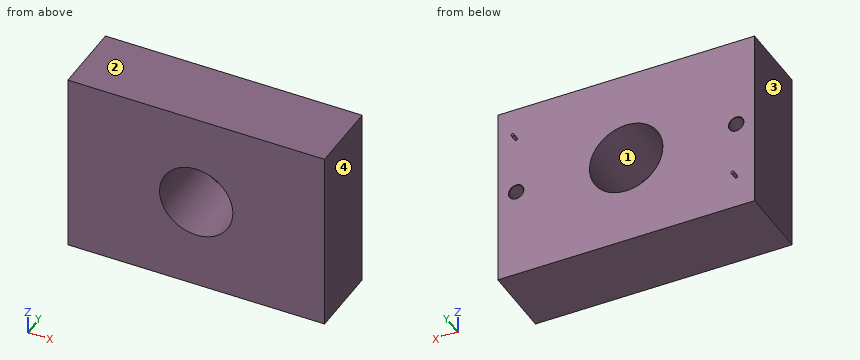
from build123d import *

# Parameters (mm, degrees)
SKETCH1_W                                      = 175
SKETCH1_H                                      = 125
SKETCH1_R                                      = 25
BOSS_EXTRUDE1_DEPTH                            = 50
SKETCH1_4_R                                    = 1
BOSS_EXTRUDE2_DEPTH                            = 5
CBORE_FOR_M12_HEX_HEAD_MACHINE_SCREW1_AT_COUNT = 2
CBORE_FOR_M12_HEX_HEAD_MACHINE_SCREW1_AT_PITCH = 150


with BuildPart() as part:
    # Sketch1 → Boss-Extrude1 (new body)
    with BuildSketch(Plane(origin=(0, 0, 0), x_dir=(1, 0, 0), z_dir=(0, 1, 0))):
        with Locations((87.5, 62.5)):
            Rectangle(SKETCH1_W, SKETCH1_H)
        with Locations(Location((87.5, 62.5, 0), (0, 0, 270))):
            Circle(SKETCH1_R, mode=Mode.SUBTRACT)
    extrude(amount=-BOSS_EXTRUDE1_DEPTH)

    # Sketch1_4 → Boss-Extrude2 (add)
    with BuildSketch(Plane(origin=(0, 0, 0), x_dir=(1, 0, 0), z_dir=(0, 1, 0))):
        with Locations(Location((12.5, 102.5, 0), (0, 0, 270))):
            Circle(SKETCH1_4_R)
        with Locations(Location((162.5, 22.5, 0), (0, 0, 270))):
            Circle(SKETCH1_4_R)
    extrude(amount=BOSS_EXTRUDE2_DEPTH)

    # Sketch5 → CBORE for M12 Hex Head Machine Screw1 (revolve, cut)
    with BuildSketch(Plane(origin=(12.5, 0, -62.5), x_dir=(0, 0, 1), z_dir=(1, 0, 0))):
        Polygon((0, 0), (0, 28), (4.25, 25.446342369), (4.25, 20), (5, 20), (5, 0.25), (5.25, 0), align=None)
    cbore_for_m12_hex_head_machine_screw1 = revolve(axis=Axis((12.5, 6.35, -62.5), (0, -1, 0)), mode=Mode.SUBTRACT)

    # CBORE for M12 Hex Head Machine Screw1 at: CBORE for M12 Hex Head Machine Screw1 ×2
    with Locations(*[(i * CBORE_FOR_M12_HEX_HEAD_MACHINE_SCREW1_AT_PITCH, 0, 0) for i in range(1, CBORE_FOR_M12_HEX_HEAD_MACHINE_SCREW1_AT_COUNT)]):
        add(cbore_for_m12_hex_head_machine_screw1, mode=Mode.SUBTRACT)


solid = part.part
Can you work these out from the model? Positions are in its coordinate system, mm. Face numbers are marked on the shaded views. Round coordinates to 2 decimals unless told otherwise and drop trailing zeros. Order: outer loops, then holes, each group sorted by start corner. A loop starts at its lowest first (then second) coordinate and runs counter-clockwise, first axis right, second up. Notation, with made-up numbers: M 40,7 L 65,7 A19 cw 65,40 Z; hole C 86.25,29.5 d5. An arc over 180 degrees is marked long. Use a Markdown table: item, result.
1) Imagine slicing it at A-A (x = 87.5). List the corners of the cut face in (y, z) for me.
Geometry says:
| item | result |
|---|---|
| outline | M -50,-125 L 0,-125 L 0,-87.5 L -50,-87.5 Z; M -50,-37.5 L 0,-37.5 L 0,0 L -50,0 Z |
2) Imagine slicing it at C-C (z = -48.5). List the corners of the cut face in (x, y) for me.
Geometry says:
| item | result |
|---|---|
| outline | M 0,-50 L 66.79,-50 L 66.79,0 L 0,0 Z; M 108.21,-50 L 175,-50 L 175,0 L 108.21,0 Z |
3) Imagine slicing it at B-B (y = -23.5). List the corners of the cut face in (x, z) for me, then the cut area to 3 significant figures.
Geometry says:
| item | result |
|---|---|
| outline | M 0,-125 L 175,-125 L 175,0 L 0,0 Z; hole C 12.5,-62.5 d8.5; hole C 87.5,-62.5 d50; hole C 162.5,-62.5 d8.5 |
| area | 19,800 mm² |
4) I'm going to push flat-ended pins straight in: P1, Ø1, axis at x = 21, z = -26.5, coming from the +Y side; P2, Ø4, axis at y = -34.5, z = -15.5, coming from the -X side; P3, Ø5, axis at x = 14.5, z = -62, coming from the +Y side. Where does each tip first touch, or does it pass through?
Geometry says:
| item | result |
|---|---|
| P1 | stops at y = 0 |
| P2 | stops at x = 0 |
| P3 | stops at y = -20 |
5) If we mould it in two halves opening along X, with no side actions, what happens to the marked faces 1, 2, 3 and 4? For each: +X half, -X half, draft (parallel to the pull), parting line (faces both ways), or undercut.
Geometry says:
| item | result |
|---|---|
| face 1 | undercut |
| face 2 | draft |
| face 3 | -X half |
| face 4 | +X half |
6) If I drill on line 1 along X through (y, z) = (-6, -62) (3 decimals); line 2 along X through (y, z) = (-22.6, -62.5); line 3 along Z through (x, y) = (87, -38) (3 decimals), over which ranges is the centre line in solid material (lowest first)?
Geometry says:
| item | result |
|---|---|
| line 1 | x = 0 to 7.525, 17.475 to 62.505, 112.495 to 157.525, 167.475 to 175 |
| line 2 | x = 0 to 8.25, 16.75 to 62.5, 112.5 to 158.25, 166.75 to 175 |
| line 3 | z = -125 to -87.495, -37.505 to 0 |
7) Imagine slicing it at D-D (y = -36). List the corners of the cut face in (x, z) for me.
Geometry says:
| item | result |
|---|---|
| outline | M 0,-125 L 175,-125 L 175,0 L 0,0 Z; hole C 87.5,-62.5 d50 |
